Here's how the part is built. I have some questions about the finished solid (model axes, mm). A direction names the side the tool comes from. Coordinates: 2 decimals unless noted, no trailing zeros. Write each loop counter-clockwise with the first axis right and the second up, starting at its lowest first coordinate (ties: lowest second). Pieces come first, ordered by that corner, then holes.
Item 1: I'm going to push flat-ended pins straight in: P1, Ø6, axis at y = -9.5, z = 43, coming from the -X side; P2, Ø1.5, axis at x = 0.5, y = 8.5, coming from the -Z side; P3, Ø1.6, axis at x = 31, z = 99, coming from the -Y side. Where does each tip first touch, or does it pass through?
Item 2: I want a section at C-C (x = -15.5). Please give me the cut outline in (y, z).
Item 3: I want a section at D-D (y = -19.5). Please give me the cut outline in (x, z).
Item 4: For faces 1 (the face through (27, 0, 17.98)), 2 (the face through (-27, 0, 17.98)), 3 (the face through (-22.5, 0, 20)), 4 (the face through (-22.5, 0, 71)), 5 (the face through (31.5, 0.07, 98.99)), which set-ups out of +Z, -Z, +X, -X, +Y, -Y let a thin tool reach every point of the face, with its end or its side?
Item 5: If we mould it in two halves opening along X, with no side actions, what happens to faces 6 (the face through (0, 0, 42.5)), 7 (the face through (28.8, 1.2, 98)), 8 (the face through (30, 0, 21))? For each: pulls with the +X half, pulls with the -X half, needs draft (parallel to the pull), parting line crosses it, or undercut.
Item 6: Please list where these lines run through material, in increasing order: line 1 (X direction, y = -4.5, z = 53.5); line 2 (Z direction, x = -11.5, y = -12); line 3 (Y direction, x = -4, z = 23.5).
Item 7: I want a section at A-A (y = 0). Count the separate pieces of the cut face and the enclosed holes in it, and give its area (4 significant figures).
Item 8: I want a section at B-B (z = 51.5). Please give me the cut outline in (x, y), and give its area (3 significant figures).
Autodesk Inventor part; units mm, degrees
ref_plane "YZ Plane" through (0, 0, 0) normal (1, 0, 0) x (0, 1, 0)
ref_plane "XZ Plane" through (0, 0, 0) normal (0, 1, 0) x (-1, 0, 0)
ref_plane "XY Plane" through (0, 0, 0) normal (0, 0, 1) x (1, 0, 0)
sketch "Boceto1" plane through (0, 0, 0) normal (0, 0, 1) x (1, 0, 0)
  line L0 (-22.5, 22.5) -> (-22.5, -22.5)
  line L1 (-22.5, -22.5) -> (22.5, -22.5)
  line L2 (22.5, -22.5) -> (22.5, 22.5)
  line L3 (-25, 22.5) -> (-25, -25)
  line L4 (-25, -25) -> (25, -25)
  line L5 (25, -25) -> (25, 22.5)
  line L6 (22.5, 22.5) -> (25, 22.5)
  line L7 (-22.5, 22.5) -> (-25, 22.5)
extrude "Extrusión1" add sketch "Boceto1" along normal blind 100
sketch "Boceto2" plane through (-22.5, -22.5, 0) normal (0, 1, 0) x (1, 0, 0)
  line L0 (-2.5, -100) -> (47.5, -100)
  line L1 (22.5, -40) -> (45, -40)
  line L2 (45, 0) -> (45, -100)
  line L3 (0, 0) -> (0, -100)
  line L4 (0, -40) -> (22.5, -40)
  line L5 (22.5, -42.5) -> (45, -42.5)
  line L6 (22.5, -42.5) -> (0, -42.5)
  line L7 (45, -40) -> (45, -42.5)
  line L8 (0, -40) -> (0, -42.5)
  point P0 (22.5, 0)
  dimension "d10" = 2.5
extrude "Extrusión2" add sketch "Boceto2" along normal blind 45 contours L3 L4 L1 L2 L5 L6
sketch "Boceto3" plane through (25, -25, 0) normal (1, 0, 0) x (0, 0, -1)
  line L0 (-100, 2.5) -> (-100, 47.5)
  line L1 (-100, 25) -> (-100, 20)
  line L2 (-100, 25) -> (-100, 30)
  line L3 (-100, 30) -> (-98, 30)
  line L4 (-98, 30) -> (-98, 20)
  line L5 (-98, 20) -> (-100, 20)
  point P0 (0, 25)
  dimension "d13" = 5
  dimension "d14" = 5
  dimension "d15" = 2
sketch "Boceto4" plane through (-25, -25, 0) normal (-1, 0, 0) x (0, 0, 1)
  line L0 (100, 2.5) -> (100, 47.5)
  line L1 (100, 25) -> (100, 20)
  line L2 (100, 25) -> (100, 30)
  line L3 (100, 30) -> (98, 30)
  line L4 (98, 30) -> (98, 20)
  line L5 (98, 20) -> (100, 20)
  point P0 (0, 25)
  dimension "d16" = 5
  dimension "d17" = 5
  dimension "d18" = 2
extrude "Extrusión3" add sketch "Boceto4" along normal blind 10
extrude "Extrusión4" add sketch "Boceto3" along normal blind 10
sketch "Boceto5" plane through (25, -5, 98) normal (0, 0, -1) x (-1, 0, 0)
  line L0 (0, 0) -> (-10, 0)
  line L1 (0, 10) -> (0, 27.5)
  line L2 (0, 10) -> (-10, 10)
  line L3 (50, 0) -> (50, -20)
  line L4 (50, 0) -> (59.9457, 0)
  line L5 (50, 27.5) -> (50, 10)
  circle A0 centre (-5, 5) radius 1.5
  circle A1 centre (54.9729, 5) radius 1.5
  point P0 (25, 5)
  dimension "d23" = 3
  dimension "d24" = 3
extrude "Extrusión5" cut sketch "Boceto5" against normal through all
sketch "Boceto7" plane through (25, -25, 0) normal (1, 0, 0) x (0, 0, -1)
  line L0 (-17.98, 25) -> (-17.98, 30)
  line L1 (-17.98, 30) -> (-17.98, 25)
  line L2 (-17.98, 25) -> (-17.98, 20)
  line L3 (-17.98, 20) -> (-22.98, 20)
  line L4 (-22.98, 20) -> (-22.98, 30)
  line L5 (-22.98, 30) -> (-17.98, 30)
  point P0 (0, 25)
  dimension "d27" = 17.98
  dimension "d28" = 5
  dimension "d29" = 5
  dimension "d30" = 5
sketch "Boceto8" plane through (-25, -25, 0) normal (-1, 0, 0) x (0, 0, 1)
  line L0 (0, 25) -> (17.98, 25)
  line L1 (17.98, 25) -> (17.98, 20)
  line L2 (17.98, 20) -> (22.98, 20)
  line L3 (22.98, 20) -> (22.98, 30)
  line L4 (22.98, 30) -> (17.98, 30)
  line L5 (17.98, 30) -> (17.98, 25)
  dimension "d31" = 17.98
  dimension "d32" = 5
  dimension "d33" = 5
  dimension "d34" = 10
  dimension "d35" = 5
  dimension "d36" = 5
extrude "Extrusión6" add sketch "Boceto8" along normal blind 5
extrude "Extrusión7" add sketch "Boceto7" along normal blind 5
properties part number "Torre Motor" material "Plástico ABS"
Answer:
1. P1: stops at x = -25
1. P2: stops at z = 40
1. P3: stops at y = -5
2. outline: (-25, 0) - (-22.5, 0) - (-22.5, 40) - (22.5, 40) - (22.5, 42.5) - (-22.5, 42.5) - (-22.5, 100) - (-25, 100) - close
3. outline: (-25, 0) - (-22.5, 0) - (-22.5, 40) - (22.5, 40) - (22.5, 0) - (25, 0) - (25, 100) - (22.5, 100) - (22.5, 42.5) - (-22.5, 42.5) - (-22.5, 100) - (-25, 100) - close
4. face 1: -Z, +X, +Y, -Y
4. face 2: -Z, -X, +Y, -Y
4. face 3: -Z, +Y
4. face 4: +Z, +Y
4. face 5: +Z
5. face 6: undercut
5. face 7: needs draft
5. face 8: pulls with the +X half
6. line 1: x = -25 to -22.5, 22.5 to 25
6. line 2: z = 40 to 42.5
6. line 3: y = -25 to -22.5
7. separate pieces: 3
7. enclosed holes: 0
7. area: 690.5 mm2
8. outline: (-25, -25) - (25, -25) - (25, 22.5) - (22.5, 22.5) - (22.5, -22.5) - (-22.5, -22.5) - (-22.5, 22.5) - (-25, 22.5) - close
8. area: 350 mm2
